Model file for the job. Use its own axes, mm. A direction names the side the tool comes from. Give positions to 0.01 mm unless a question says otherwise; leave off trailing zeros. Loops run counter-clockwise (first coordinate to the right, second up) from the corner with the lowest first, then second, coordinate; pieces in that order, holes last. Notation, with made-up numbers: (19.5, 15.25) - (51.5, 15.25) arc R26 cw to (51.5, 30.25) - close; hole circle Ø5 at (32.5, 68.5). An arc over 180 degrees is marked (long way). Use a Markdown table: item, result.
from build123d import *

# Parameters (mm, degrees)
F0_W     = 16
F0_H     = 92
F0_R     = 2.5
F1_DEPTH = 5
F3_DEPTH = 13
F2_W     = 3
F2_H     = 72
F4_DEPTH = 5
F5_R     = 2
F6_DEPTH = 25


with BuildPart() as f1:
    # F0 (on Top) → F1 (new body)
    with BuildSketch(Plane.XY):
        Rectangle(F0_W, F0_H)
        with Locations((4.5, -20)):
            Circle(F0_R, mode=Mode.SUBTRACT)
        with Locations((4.5, 17.5)):
            Circle(F0_R, mode=Mode.SUBTRACT)
    extrude(amount=F1_DEPTH)

    # F2 (on face) → F3 (join)
    with BuildSketch(Plane.XY.offset(5)):
        Polygon((-5, -36), (-8, -36), (-8, -46), (8, -46), (8, -36), align=None)
        Polygon((8, 46), (-8, 46), (-8, 36), (-5, 36), (8, 36), align=None)
    extrude(amount=F3_DEPTH)

    # F2 (on face) → F4 (join)
    with BuildSketch(Plane.XY.offset(5)):
        Polygon((8, 46), (-8, 46), (-8, 36), (-5, 36), (8, 36), align=None)
        with Locations((-6.5, 0)):
            Rectangle(F2_W, F2_H)
        Polygon((-5, -36), (-8, -36), (-8, -46), (8, -46), (8, -36), align=None)
    extrude(amount=F4_DEPTH)

    # F5 (on face) → F6 (cut)
    with BuildSketch(Plane(origin=(0, 0, 0), x_dir=(1, 0, 0), z_dir=(0, 0, -1))):
        with Locations((-3.5, -41)):
            Circle(F5_R)
        with Locations((-3.5, 41)):
            Circle(F5_R)
    extrude(amount=-F6_DEPTH, mode=Mode.SUBTRACT)


solid = f1.part
(1) Pin check, flat tips, straight feed: P1, Ø0.9, axis at x = -7, y = -15.5, coming from the +Z side; P2, Ø6, axis at x = 3, y = -5, coming from the +Z side. Stop position of each tip, or through.
Computed:
| item | result |
|---|---|
| P1 | z = 10 |
| P2 | z = 5 |
(2) 3-axis set-ups, long thin cutter, end or side, ignore diameter. For faces 1 (the flat face through (-5, -1, 7)), 2 (the flat face through (0, -41, 18)), 3 (the flat face through (-7, 1, 10)): which of +Z, -Z, +X, -X, +Y, -Y reach the whole face in a straight line?
Computed:
| item | result |
|---|---|
| face 1 | +Z, +X |
| face 2 | +Z, +X, -X, +Y, -Y |
| face 3 | +Z, +X, -X |
(3) Drill centre lines: probe 1 along Y at (x, z) = (4.5, 2.35); probe 2 along Y at (x, z) = (-3.25, 1.75); probe 3 along Y at (x, z) = (1.75, 16.5). Where is each one in solid material? Low to high. Write a range as [from, to].
Computed:
| item | result |
|---|---|
| probe 1 | [-46, -22.5], [-17.5, 15], [20, 46] |
| probe 2 | [-46, -42.98], [-39.02, 39.02], [42.98, 46] |
| probe 3 | [-46, -36], [36, 46] |
(4) Slice it at C-C, the plane y = 17.5. Write the cut outline in (x, z).
Computed:
| item | result |
|---|---|
| outline | (-8, 0) - (2, 0) - (2, 5) - (-5, 5) - (-5, 10) - (-8, 10) - close; (7, 0) - (8, 0) - (8, 5) - (7, 5) - close |
(5) Slice it at A-A, the plane x = -3.5. Write the cut outline in (y, z).
Computed:
| item | result |
|---|---|
| outline | (-46, 0) - (-43, 0) - (-43, 18) - (-46, 18) - close; (-39, 0) - (39, 0) - (39, 18) - (36, 18) - (36, 5) - (-36, 5) - (-36, 18) - (-39, 18) - close; (43, 0) - (46, 0) - (46, 18) - (43, 18) - close |
(6) Mould opens along Y. For faces 4 (the flat face through (1, 1, 5)), 5 (the flat face through (0, 46, 9)), 6 (the flat face through (0, -46, 9)) say: pulls with the +Y half, pulls with the -Y half, needs draft (parallel to the pull), parting line crosses it, or undercut.
Computed:
| item | result |
|---|---|
| face 4 | undercut |
| face 5 | pulls with the +Y half |
| face 6 | pulls with the -Y half |
(7) Slice it at D-D, the plane z = 1.25. Write the cut outline in (x, y), plus the area to 3 significant figures.
Computed:
| item | result |
|---|---|
| outline | (-8, -46) - (8, -46) - (8, 46) - (-8, 46) - close; hole circle Ø4 at (-3.5, -41); hole circle Ø4 at (-3.5, 41); hole circle Ø5 at (4.5, -20); hole circle Ø5 at (4.5, 17.5) |
| area | 1,410 mm² |
(8) Slice it at B-B, the plane z = 14. Write the cut outline in (x, y).
Computed:
| item | result |
|---|---|
| outline | (-8, -46) - (8, -46) - (8, -36) - (-8, -36) - close; (-8, 36) - (8, 36) - (8, 46) - (-8, 46) - close; hole circle Ø4 at (-3.5, -41); hole circle Ø4 at (-3.5, 41) |
